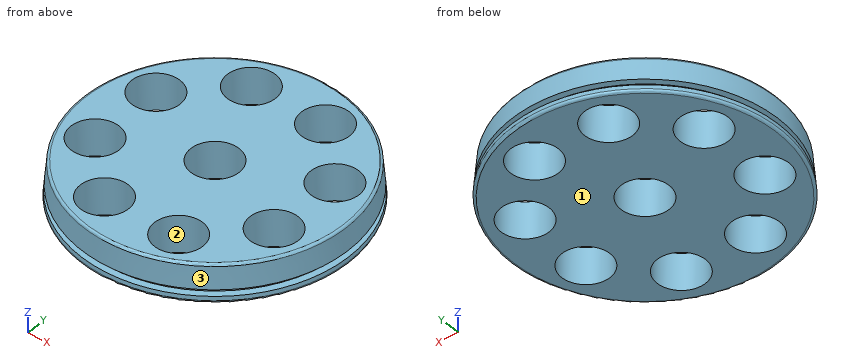
from build123d import *

# Parameters (mm, degrees)
SKETCH1_R           = 69.85
BOSS_EXTRUDE1_DEPTH = 19.05
BOSS_EXTRUDE1_TAPER = 5
FILLET2_R           = 1.27
SKETCH3_R           = 12.573
CUT_EXTRUDE1_DEPTH  = 19.05


with BuildPart() as part:
    # Sketch1 → Boss-Extrude1 (new body)
    with BuildSketch(Plane.XY):
        Circle(SKETCH1_R)
    extrude(amount=BOSS_EXTRUDE1_DEPTH, taper=BOSS_EXTRUDE1_TAPER)

    # Fillet2
    fillet2_edges = [part.edges().sort_by_distance(p)[0] for p in [
        (-69.85, 0, 0),
        (-68.18334096, 0, 19.05),
    ]]
    fillet(fillet2_edges, radius=FILLET2_R)

    # Sketch2 → Cut-Revolve1 (revolve, cut)
    with BuildSketch(Plane(origin=(0, 0, 0), x_dir=(1, 0, 0), z_dir=(0, 1, 0))):
        Polygon((-66.369445843, -3.770276507), (-66.369445843, -6.389723493), (-69.544445843, -6.6675), (-69.544445843, -3.4925), align=None)
    revolve(axis=Axis((0, 0, 0), (0, 0, 1)), mode=Mode.SUBTRACT)

    # Sketch3 → Cut-Extrude1 (cut)
    with BuildSketch(Plane(origin=(0, 0, 0), x_dir=(-1, 0, 0), z_dir=(0, 0, -1))):
        with Locations((-19.440318364, 46.933080252)):
            Circle(SKETCH3_R)
        with Locations((19.440318364, 46.933080252)):
            Circle(SKETCH3_R)
        with Locations((46.933080252, 19.440318364)):
            Circle(SKETCH3_R)
        with Locations((46.933080252, -19.440318364)):
            Circle(SKETCH3_R)
        with Locations((19.440318364, -46.933080252)):
            Circle(SKETCH3_R)
        with Locations((-19.440318364, -46.933080252)):
            Circle(SKETCH3_R)
        with Locations((-46.933080252, -19.440318364)):
            Circle(SKETCH3_R)
        with Locations((-46.933080252, 19.440318364)):
            Circle(SKETCH3_R)
        Circle(SKETCH3_R)
    extrude(amount=-CUT_EXTRUDE1_DEPTH, mode=Mode.SUBTRACT)


solid = part.part
Geometry check sheet. Reference: the model listing, model coordinates, mm. Face numbers are marked on the shaded views. Give positions to 0.01 mm unless a question says otherwise; leave off trailing zeros. Order: outer loops, then holes, each group sorted by start corner. A loop starts at its lowest first (then second) coordinate and runs counter-clockwise, first axis right, second up. Notation, with made-up numbers: (26.25, -10) - (43.25, -10) arc R26 cw to (43.25, 24) - close; hole circle Ø7 at (65, 53.5). An arc over 180 degrees is marked (long way). Answer as a JSON object with one key per item and string values.
(1) Material ranges on line 1 (Z direction, x = 61.5, y = -25.5); line 2 (Y direction, x = -39.5, z = 9); line 3 (X direction, y = 37, z = 5.75), recorded low to high.
Report:
{"line 1": "0 to 3.75, 6.41 to 19.05", "line 2": "-56.65 to -29.58, -9.3 to 9.3, 29.58 to 56.65", "line 3": "-55.1 to -27.15, -11.73 to 11.73, 27.15 to 55.1"}
(2) Cross-section at C-C (z = 12). State how many separate pieces and enclosed holes the cut face has, then the cut area to 3 significant figures.
Report:
{"separate pieces": "1", "enclosed holes": "9", "area": "10,400 mm^2"}
(3) Depth check by flat-ended pin: pin 1 Ø3 at (x, z) = (44.5, 7.5) entering from -Y; pin 2 Ø8 at (y, z) = (7, 13.5) entering from -X; pin 3 Ø1.5 at (y, z) = (-17.5, 8.5) entering from -X. Enter the tip coordinate at first touch or a pass-through.
Report:
{"pin 1": "y = -54.22", "pin 2": "x = -68.8", "pin 3": "x = -67.06"}
(4) Cross-section at A-A (y = 0). Record the cut outline in (x, z).
Report:
{"outline": "(-69.73, 1.38) arc R1.27 ccw to (-68.46, 0) - (-12.57, 0) - (-12.57, 19.05) - (-67.02, 19.05) arc R1.27 ccw to (-68.28, 17.89) - (-69.27, 6.64) - (-66.37, 6.39) - (-66.37, 3.77) - (-69.54, 3.49) - close; (12.57, 0) - (68.46, 0) arc R1.27 ccw to (69.73, 1.38) - (69.54, 3.49) - (66.37, 3.77) - (66.37, 6.39) - (69.27, 6.64) - (68.28, 17.89) arc R1.27 ccw to (67.02, 19.05) - (12.57, 19.05) - close"}
(5) Draft check along Y on the marked faces 1, 2 and 3. Enter one of: released by +Y, released by -Y, zero draft, split by the parting line, or undercut.
Report:
{"face 1": "zero draft", "face 2": "undercut", "face 3": "split by the parting line"}
